```python
from build123d import *

# Parameters (mm, degrees)
CUT_EXTRUDE_1_REACH = 117.678
SKETCH_2_R          = 17
SKETCH_3_R          = 9
CUT_EXTRUDE_2_DEPTH = 35


with BuildPart() as part:
    # 草图1 → 旋转1 (revolve)
    with BuildSketch(Plane.XY, mode=Mode.PRIVATE) as revolve_1_sk:
        Polygon((63, 0), (63, 26), (26, 26), (26, 37), (27, 37), (27, 39), (22, 39), (22, 58), (27, 58), (27, 60), (26, 60), (26, 94), (36, 94), (36, 91.414213562), (34.585786438, 90), (36, 88.585786438), (37.414213562, 90), (38.5, 90), (38.5, 61), (65, 61), (65, 43), (69.5, 38.5), (69.5, 0), align=None)
    revolve(revolve_1_sk.sketch.rotate(Axis((0, 19.246271831, 0), (0, -1, 0)), 90), axis=Axis((0, 19.246271831, 0), (0, -1, 0)))

    # 切除-拉伸1: up to this face of the body (flat: up to its plane)
    cut_extrude_1_end = Plane(part.part.faces().sort_by_distance((0, 94, -27.018233765))[0])
    # 草图2 → 切除-拉伸1 (cut, up to the picked face)
    with BuildSketch(Plane(origin=(0, 61, 0), x_dir=(1, 0, 0), z_dir=(0, 1, 0)), mode=Mode.PRIVATE) as cut_extrude_1_sk1:
        with Locations((-48.75, 0)):
            Circle(SKETCH_2_R)
    cut_extrude_1_tool1 = split(extrude(cut_extrude_1_sk1.sketch, amount=CUT_EXTRUDE_1_REACH, mode=Mode.PRIVATE), bisect_by=cut_extrude_1_end, keep=Keep.BOTH, mode=Mode.PRIVATE)
    # 草图2 → 切除-拉伸1 (cut, up to the picked face)
    with BuildSketch(Plane(origin=(0, 61, 0), x_dir=(1, 0, 0), z_dir=(0, 1, 0)), mode=Mode.PRIVATE) as cut_extrude_1_sk2:
        with Locations((24.375, 42.218738434)):
            Circle(SKETCH_2_R)
    cut_extrude_1_tool2 = split(extrude(cut_extrude_1_sk2.sketch, amount=CUT_EXTRUDE_1_REACH, mode=Mode.PRIVATE), bisect_by=cut_extrude_1_end, keep=Keep.BOTH, mode=Mode.PRIVATE)
    # 草图2 → 切除-拉伸1 (cut, up to the picked face)
    with BuildSketch(Plane(origin=(0, 61, 0), x_dir=(1, 0, 0), z_dir=(0, 1, 0)), mode=Mode.PRIVATE) as cut_extrude_1_sk3:
        with Locations((24.375, -42.218738434)):
            Circle(SKETCH_2_R)
    cut_extrude_1_tool3 = split(extrude(cut_extrude_1_sk3.sketch, amount=CUT_EXTRUDE_1_REACH, mode=Mode.PRIVATE), bisect_by=cut_extrude_1_end, keep=Keep.BOTH, mode=Mode.PRIVATE)
    add(cut_extrude_1_tool1.solids().sort_by(Axis((-48.75, 61, 0), (0, 1, 0)))[0], mode=Mode.SUBTRACT)
    add(cut_extrude_1_tool2.solids().sort_by(Axis((24.375, 61, -42.218738), (0, 1, 0)))[0], mode=Mode.SUBTRACT)
    add(cut_extrude_1_tool3.solids().sort_by(Axis((24.375, 61, 42.218738), (0, 1, 0)))[0], mode=Mode.SUBTRACT)

    # 草图3 → 切除-拉伸2 (cut)
    with BuildSketch(Plane(origin=(0, 61, 0), x_dir=(1, 0, 0), z_dir=(0, 1, 0))):
        with Locations(Location((24.375, 42.218738434, 0), (0, 0, 270))):
            Circle(SKETCH_3_R)
        with Locations(Location((24.375, -42.218738434, 0), (0, 0, 270))):
            Circle(SKETCH_3_R)
        with Locations(Location((-48.75, 0, 0), (0, 0, 270))):
            Circle(SKETCH_3_R)
    extrude(amount=-CUT_EXTRUDE_2_DEPTH, mode=Mode.SUBTRACT)


solid = part.part
```
Design review of the part built by this model. Coordinates are the model's own, in mm. A direction names the side the tool comes from. Round coordinates to 2 decimals unless told otherwise and drop trailing zeros. Write each loop counter-clockwise with the first axis right and the second up, starting at its lowest first coordinate (ties: lowest second). Pieces come first, ordered by that corner, then holes. Notation, with made-up numbers: (-20.5, 56.5) -> (6.5, 56.5) arc R5 cw to (6.5, 65.5) -> close; hole circle Ø5 at (71, 40.25). An arc over 180 degrees is marked (long way). Write item = value, one per line. Start each with the question number.
1) Tool access review of faces 1 (the face through (20, 58, 10)), 2 (the face through (-19.52, 51.87, 62)), 3 (the face through (-62.464, 13.182, -8.201)): name each direction out of +Z, -Z, +X, -X, +Y, -Y from which nothing blocks a thin tool from reaching the whole face with its end or side.
2) Take a section at D-D, the plane y = 23. State the section outline as (x, z) points, plus the area to 3 significant figures.
3) Clearance check with flat-ended pins moving along their axes: pin 1 (6 mm diameter, centred on y = 77.5, z = -26.5, fed in from +X); pin 2 (8 mm diameter, centred on y = 67, z = -41.5, fed in from +X); pin 3 (1.5 mm diameter, centred on x = 25, y = 54, fed in from +Z). State where each tip first meets the part, or that it passes through.
4) Take a section at B-B, the plane z = 0. Count the separate pieces of the cut face and the enclosed holes in it, plus the area to 3 significant figures.
5) Wall thickness on probe 1 along X at (y, z) = (48, 0); probe 2 along X at (y, z) = (29.5, 0); probe 3 along X at (y, z) = (20.25, 0): over which ranges is each line inside the solid? List them lowest first. Write a range as from..to.
6) Mouldability with a two-part tool opening along Z and no side actions: class faces 4 (the face through (24, 94, 11)), 5 (the face through (24.77, 43.74, -51.21)), 6 (the face through (-18.907, 75.297, 33.538)), 7 (the face through (-19.609, 42.718, 62.267)) as +Z half, -Z half, draft (parallel to the pull), parting line (faces both ways), or undercut.
7) Take a section at A-A, the plane y = 74.5. State the section outline as (x, z) points (3 decimals).
8) Take a section at C-C, the plane y = 34.5. State the section outline as (x, z) points (3 decimals), plus the area to 3 significant figures.
Results list:
q1.face_1 = none
q1.face_2 = +Y
q1.face_3 = -Y
q2.outline = circle Ø139 at (0, 0); hole circle Ø126 at (0, 0)
q2.area = 2,710 mm²
q3.pin_1 = 30.5
q3.pin_2 = 8.04
q3.pin_3 = 60.31
q4.separate_pieces = 3
q4.enclosed_holes = 0
q4.area = 3,300 mm²
q5.probe_1 = -65..-57.75, -39.75..-22, 22..65
q5.probe_2 = -69.5..-57.75, -39.75..-26, 26..69.5
q5.probe_3 = -69.5..-63, 63..69.5
q6.face_4 = draft
q6.face_5 = undercut
q6.face_6 = +Z half
q6.face_7 = parting line
q7.outline = (-36.613, -11.904) arc R38.5 ccw to (7.998, -37.66) arc R17 cw to (28.616, -25.756) arc R38.5 ccw to (28.616, 25.756) arc R17 cw to (7.998, 37.66) arc R38.5 ccw to (-36.613, 11.904) arc R17 cw to start; hole circle Ø52 at (0, 0)
q8.outline = circle Ø139 at (0, 0); hole circle Ø18 at (-48.75, 0); hole circle Ø52 at (0, 0); hole circle Ø18 at (24.375, -42.219); hole circle Ø18 at (24.375, 42.219)
q8.area = 12,300 mm²
